Autodesk Inventor part; units mm, degrees
ref_plane "YZ Plane" through (0, 0, 0) normal (1, 0, 0) x (0, 1, 0)
ref_plane "XZ Plane" through (0, 0, 0) normal (0, 1, 0) x (-1, 0, 0)
ref_plane "XY Plane" through (0, 0, 0) normal (0, 0, 1) x (1, 0, 0)
ref_plane "Work Plane1" through (-80.5192, 95.2728, -37.0091) normal (-0.0000001, -1, 0.0000001) x (1, -0.0000001, 0)
sketch "Sketch1" plane through (-80.5192, 95.2728, -37.0091) normal (-0.0000001, -1, 0.0000001) x (1, -0.0000001, 0)
  circle A0 centre (0, 0) radius 25
  circle A1 centre (0, 0) radius 7.5
  circle A2 centre (8.75, -15.1554) radius 2.75
  circle A3 centre (8.75, 15.1554) radius 2.75
  circle A4 centre (-17.5, 0) radius 2.75
  line L0 (8.75, 15.1554) -> (0, 0)
  line L1 (0, 0) -> (8.75, -15.1554)
  line L2 (0, 0) -> (-17.5, 0)
  point P0 (80.5192, 37.0091)
  dimension "d0" = 50
  dimension "d1" = 15
extrude "Extrusion1" add sketch "Sketch1" along normal blind 30
properties part number "Pierścień"
Geometry check sheet. Reference: the model listing, model coordinates, mm. Give positions to 0.01 mm unless a question says otherwise; leave off trailing zeros. Use a Markdown table: item, result.
Q1. Section check A-A, the plane x = -72. Give the number of separate pieces and of enclosed holes in the cut face, then the cut area to 3 significant figures.
Computed:
| item | result |
|---|---|
| separate pieces | 3 |
| enclosed holes | 0 |
| area | 1,080 mm² |
Q2. Draft check along X on faces 1 (the face through (-69.146, 80.483, -22.68)), 2 (the face through (-86.4, 65.273, -42.2)), 3 (the face through (-96.5, 80.5, -39.3)), 4 (the face through (-100.36, 80.48, -21.8)). Enter one of: pulls with the +X half, pulls with the -X half, needs draft (parallel to the pull), parting line crosses it, or undercut.
Computed:
| item | result |
|---|---|
| face 1 | undercut |
| face 2 | needs draft |
| face 3 | undercut |
| face 4 | parting line crosses it |
Q3. Go/stop test with flat-tipped pins: P1, Ø2, axis at x = -98.5, y = 72.5, coming from the +Z side; P2, Ø8, axis at y = 81.5, z = -42, coming from the +X side; P3, Ø4, axis at x = -82, y = 84.5, coming from the +Z side; P4, Ø5, axis at x = -98.02, z = -37.01, coming from the +Y side. Record where each tip stops, or that it passes through.
Computed:
| item | result |
|---|---|
| P1 | stops at z = -18.66 |
| P2 | stops at x = -55.54 |
| P3 | stops at z = -12.01 |
| P4 | passes through |
Q4. Thickness scan on L1, parallel to X at y = 69, z = -36; L2, parallel to Z at x = -79.5, y = 69.5; L3, parallel to Z at x = -70, y = 79.5. Record the ranges inside material, lowest first. Write a range as [from, to].
Computed:
| item | result |
|---|---|
| L1 | x = [-105.5, -100.58], [-95.46, -87.95], [-73.09, -55.54] |
| L2 | z = [-61.99, -44.44], [-29.58, -12.03] |
| L3 | z = [-59.69, -54.27], [-50.06, -23.96], [-19.75, -14.33] |
